Work out the finished part from the listing and answer in its coordinate system (mm). Face numbers are marked on the shaded views. Round coordinates to 2 decimals unless told otherwise and drop trailing zeros. Order: outer loops, then holes, each group sorted by start corner. A loop starts at its lowest first (then second) coordinate and runs counter-clockwise, first axis right, second up. Notation, with made-up numbers: M 67,33.5 L 78,33.5 A25 cw 78,68.5 Z; hole C 77,-5.75 d6. An arc over 180 degrees is marked long. Return JSON: item names as keys, results as strings.
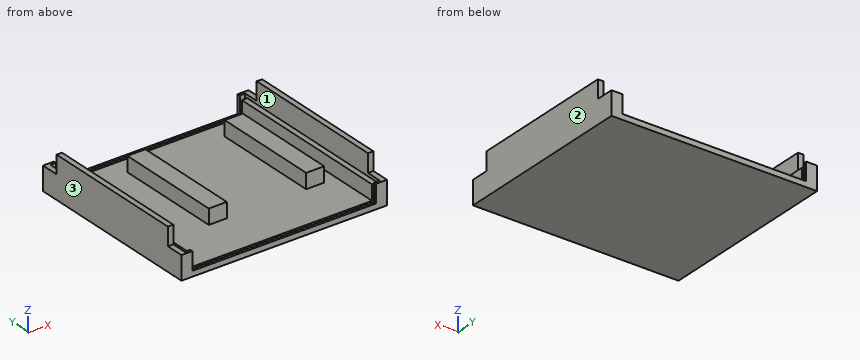
from build123d import *

# Parameters (mm, degrees)
SKETCH_W        = 114
SKETCH_H        = 102
PAD_DEPTH       = 3
SKETCH001_W     = 6
SKETCH001_H     = 102
PAD001_DEPTH    = 10
SKETCH002_W     = 3
SKETCH002_H     = 96
POCKET_DEPTH    = 1.7
SKETCH003_W     = 6
SKETCH003_H     = 102
PAD002_DEPTH    = 10
SKETCH004_W     = 3
SKETCH004_H     = 96
POCKET001_DEPTH = 1.7
SKETCH006_W     = 1.5
SKETCH006_H     = 10
POCKET002_DEPTH = 3
SKETCH007_W     = 1.5
SKETCH007_H     = 10
POCKET003_DEPTH = 3
SKETCH008_W     = 1.5
SKETCH008_H     = 10
POCKET004_DEPTH = 3
SKETCH009_W     = 1.5
SKETCH009_H     = 10
POCKET005_DEPTH = 3
SKETCH010_W     = 3
SKETCH010_H     = 82
PAD003_DEPTH    = 10
SKETCH011_W     = 3
SKETCH011_H     = 82
PAD004_DEPTH    = 10
SKETCH012_W     = 10
SKETCH012_H     = 60
PAD005_DEPTH    = 8.3
SKETCH013_W     = 10
SKETCH013_H     = 60
PAD006_DEPTH    = 8.3
SKETCH014_W     = 102
SKETCH014_H     = 1.5
POCKET006_DEPTH = 1.5
SKETCH015_W     = 102
SKETCH015_H     = 1.5
POCKET007_DEPTH = 1.5
SKETCH016_W     = 3
SKETCH016_H     = 1.5
POCKET008_DEPTH = 1.5
SKETCH017_W     = 3
SKETCH017_H     = 1.5
POCKET009_DEPTH = 1.5
SKETCH018_W     = 3
SKETCH018_H     = 1.5
POCKET010_DEPTH = 1.5
SKETCH019_W     = 3
SKETCH019_H     = 1.5
POCKET011_DEPTH = 1.5


with BuildPart() as part:
    # Sketch → Pad (new body)
    with BuildSketch(Plane.XY):
        with Locations((57, -51)):
            Rectangle(SKETCH_W, SKETCH_H)
    extrude(amount=PAD_DEPTH)

    # Sketch001 (on Face6 of Pad) → Pad001 (join)
    with BuildSketch(Plane.XY.offset(3)):
        with Locations((3, -51)):
            Rectangle(SKETCH001_W, SKETCH001_H)
    extrude(amount=PAD001_DEPTH)

    # Sketch002 (on Face10 of Pad001) → Pocket (cut)
    with BuildSketch(Plane.XY.offset(13)):
        with Locations((4.5, -51)):
            Rectangle(SKETCH002_W, SKETCH002_H)
    extrude(amount=-POCKET_DEPTH, mode=Mode.SUBTRACT)

    # Sketch003 (on Face6 of Pocket) → Pad002 (join)
    with BuildSketch(Plane.XY.offset(3)):
        with Locations((111, -51)):
            Rectangle(SKETCH003_W, SKETCH003_H)
    extrude(amount=PAD002_DEPTH)

    # Sketch004 (on Face14 of Pad002) → Pocket001 (cut)
    with BuildSketch(Plane.XY.offset(13)):
        with Locations((109.5, -51)):
            Rectangle(SKETCH004_W, SKETCH004_H)
    extrude(amount=-POCKET001_DEPTH, mode=Mode.SUBTRACT)

    # Sketch006 (on Face11 of Pocket001) → Pocket002 (cut)
    with BuildSketch(Plane.YZ.offset(6)):
        with Locations((-2.25, 8)):
            Rectangle(SKETCH006_W, SKETCH006_H)
    extrude(amount=-POCKET002_DEPTH, mode=Mode.SUBTRACT)

    # Sketch007 (on Face15 of Pocket002) → Pocket003 (cut)
    with BuildSketch(Plane.YZ.offset(6)):
        with Locations((-99.75, 8)):
            Rectangle(SKETCH007_W, SKETCH007_H)
    extrude(amount=-POCKET003_DEPTH, mode=Mode.SUBTRACT)

    # Sketch008 (on Face13 of Pocket003) → Pocket004 (cut)
    with BuildSketch(Plane(origin=(108, 0, 0), x_dir=(0, -1, 0), z_dir=(-1, 0, 0))):
        with Locations((2.25, 8)):
            Rectangle(SKETCH008_W, SKETCH008_H)
    extrude(amount=-POCKET004_DEPTH, mode=Mode.SUBTRACT)

    # Sketch009 (on Face15 of Pocket004) → Pocket005 (cut)
    with BuildSketch(Plane(origin=(108, 0, 0), x_dir=(0, -1, 0), z_dir=(-1, 0, 0))):
        with Locations((99.75, 8)):
            Rectangle(SKETCH009_W, SKETCH009_H)
    extrude(amount=-POCKET005_DEPTH, mode=Mode.SUBTRACT)

    # Sketch010 (on Face12 of Pocket005) → Pad003 (join)
    with BuildSketch(Plane.XY.offset(13)):
        with Locations((1.5, -51)):
            Rectangle(SKETCH010_W, SKETCH010_H)
    extrude(amount=PAD003_DEPTH)

    # Sketch011 (on Face22 of Pad003) → Pad004 (join)
    with BuildSketch(Plane.XY.offset(13)):
        with Locations((112.5, -51)):
            Rectangle(SKETCH011_W, SKETCH011_H)
    extrude(amount=PAD004_DEPTH)

    # Sketch012 (on Face6 of Pad004) → Pad005 (join)
    with BuildSketch(Plane.XY.offset(3)):
        with Locations((96, -43)):
            Rectangle(SKETCH012_W, SKETCH012_H)
    extrude(amount=PAD005_DEPTH)

    # Sketch013 (on Face6 of Pad005) → Pad006 (join)
    with BuildSketch(Plane.XY.offset(3)):
        with Locations((42, -43)):
            Rectangle(SKETCH013_W, SKETCH013_H)
    extrude(amount=PAD006_DEPTH)

    # Sketch014 (on Face6 of Pad006) → Pocket006 (cut)
    with BuildSketch(Plane.XY.offset(3)):
        with Locations((57, -99.75)):
            Rectangle(SKETCH014_W, SKETCH014_H)
    extrude(amount=-POCKET006_DEPTH, mode=Mode.SUBTRACT)

    # Sketch015 (on Face6 of Pocket006) → Pocket007 (cut)
    with BuildSketch(Plane.XY.offset(3)):
        with Locations((57, -2.25)):
            Rectangle(SKETCH015_W, SKETCH015_H)
    extrude(amount=-POCKET007_DEPTH, mode=Mode.SUBTRACT)

    # Sketch016 (on Face57 of Pocket007) → Pocket008 (cut)
    with BuildSketch(Plane.XY.offset(3)):
        with Locations((4.5, -99.75)):
            Rectangle(SKETCH016_W, SKETCH016_H)
    extrude(amount=-POCKET008_DEPTH, mode=Mode.SUBTRACT)

    # Sketch017 (on Face45 of Pocket008) → Pocket009 (cut)
    with BuildSketch(Plane.XY.offset(3)):
        with Locations((4.5, -2.25)):
            Rectangle(SKETCH017_W, SKETCH017_H)
    extrude(amount=-POCKET009_DEPTH, mode=Mode.SUBTRACT)

    # Sketch018 (on Face60 of Pocket009) → Pocket010 (cut)
    with BuildSketch(Plane.XY.offset(3)):
        with Locations((109.5, -99.75)):
            Rectangle(SKETCH018_W, SKETCH018_H)
    extrude(amount=-POCKET010_DEPTH, mode=Mode.SUBTRACT)

    # Sketch019 (on Face49 of Pocket010) → Pocket011 (cut)
    with BuildSketch(Plane.XY.offset(3)):
        with Locations((109.5, -2.25)):
            Rectangle(SKETCH019_W, SKETCH019_H)
    extrude(amount=-POCKET011_DEPTH, mode=Mode.SUBTRACT)


solid = part.part
Item 1: The mould has two halves that part along X. Classify the marked faces 1, 2 and 3: pulls with the +X half, pulls with the -X half, needs draft (parallel to the pull), parting line crosses it, or undercut.
Output:
{"face 1": "undercut", "face 2": "pulls with the +X half", "face 3": "pulls with the -X half"}
Item 2: Find section A-A (z = 10). State how many separate pieces and enclosed holes the cut face has, plus the area to 3 significant figures.
Output:
{"separate pieces": "4", "enclosed holes": "0", "area": "2,410 mm^2"}
Item 3: Each of these flat-tipped pins is pushed along its axis until it touches: pin 1 (2 mm diameter, centred on x = 18, y = -61.5, fed in from -Z); pin 2 (1.2 mm diameter, centred on x = 37.5, y = -101, fed in from +Z); pin 3 (3 mm diameter, centred on x = 110.5, y = -6, fed in from +Z); pin 4 (4 mm diameter, centred on x = 100, z = 12.5, fed in from -Y). Where does it stop, or does it pass through?
Output:
{"pin 1": "stops at z = 0", "pin 2": "stops at z = 3", "pin 3": "stops at z = 13", "pin 4": "stops at y = -73"}
Item 4: Find section B-B (x = 68.5). Determine the outline of the cut face in (y, z), plus the area to 4 significant figures.
Output:
{"outline": "M -102,0 L 0,0 L 0,3 L -1.5,3 L -1.5,1.5 L -3,1.5 L -3,3 L -99,3 L -99,1.5 L -100.5,1.5 L -100.5,3 L -102,3 Z", "area": "301.5 mm^2"}
Item 5: Consider line 1 along X through (y, z) = (-70, 7.5); line 2 along Y through (x, z) = (48, 2.5); line 3 along X through (y, z) = (-19.5, 18.5). Determine where each line is inside the solid, lowest interval first. Write a range as [from, to].
Output:
{"line 1": "x = [0, 6], [37, 47], [91, 101], [108, 114]", "line 2": "y = [-102, -100.5], [-99, -3], [-1.5, 0]", "line 3": "x = [0, 3], [111, 114]"}
Item 6: Find section C-C (y = -65). Determine the outline of the cut face in (x, z).
Output:
{"outline": "M 0,0 L 114,0 L 114,23 L 111,23 L 111,11.3 L 108,11.3 L 108,3 L 101,3 L 101,11.3 L 91,11.3 L 91,3 L 47,3 L 47,11.3 L 37,11.3 L 37,3 L 6,3 L 6,11.3 L 3,11.3 L 3,23 L 0,23 Z"}
Item 7: Find section D-D (x = 99). Determine the outline of the cut face in (y, z).
Output:
{"outline": "M -102,0 L 0,0 L 0,3 L -1.5,3 L -1.5,1.5 L -3,1.5 L -3,3 L -13,3 L -13,11.3 L -73,11.3 L -73,3 L -99,3 L -99,1.5 L -100.5,1.5 L -100.5,3 L -102,3 Z"}
